```python
from build123d import *

# Parameters (mm, degrees)
SKETCH2_W          = 61.210230612
SKETCH2_H          = 60
EXTRUDE1_DEPTH     = 8
CHAMFER1_SIZE      = 5
SKETCH3_R          = 12
SKETCH3_R_2        = 2.5
CUT_EXTRUDE1_DEPTH = 53.63316445


with BuildPart() as part:
    # Sketch2 → Extrude1 (new body)
    with BuildSketch(Plane(origin=(0, 0, 0), x_dir=(1, 0, 0), z_dir=(0, 1, 0))):
        with Locations((11.894884694, 0)):
            Rectangle(SKETCH2_W, SKETCH2_H)
    extrude(amount=EXTRUDE1_DEPTH)

    # Chamfer1
    chamfer1_edges = [part.edges().sort_by_distance(p)[0] for p in [
        (-18.710230612, 4, 30),
        (-18.710230612, 4, -30),
    ]]
    chamfer(chamfer1_edges, length=CHAMFER1_SIZE)

    # Sketch3 → Cut-Extrude1 (cut, through all)
    with BuildSketch(Plane(origin=(0, 8, 0), x_dir=(1, 0, 0), z_dir=(0, 1, 0))):
        with Locations(Location((12, 0, 0), (0, 0, 270))):
            Circle(SKETCH3_R)
        with Locations(Location((-11.57, 23.57, 0), (0, 0, 270))):
            Circle(SKETCH3_R_2)
        with Locations(Location((35.57, 23.57, 0), (0, 0, 270))):
            Circle(SKETCH3_R_2)
        with Locations(Location((-11.57, -23.57, 0), (0, 0, 270))):
            Circle(SKETCH3_R_2)
        with Locations(Location((35.57, -23.57, 0), (0, 0, 270))):
            Circle(SKETCH3_R_2)
    extrude(amount=-CUT_EXTRUDE1_DEPTH, mode=Mode.SUBTRACT)


solid = part.part
```
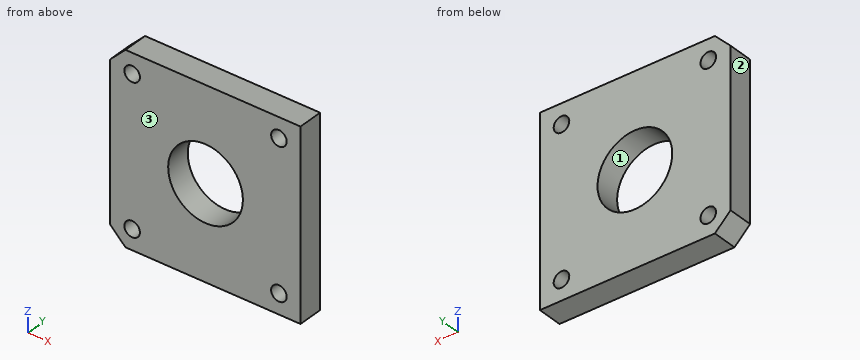
Can you work these out from the model? Positions are in its coordinate system, mm. Face numbers are marked on the shaded views. Coordinates: 2 decimals unless noted, no trailing zeros. Write each loop counter-clockwise with the first axis right and the second up, starting at its lowest first coordinate (ties: lowest second). Pieces come first, ordered by that corner, then holes. Notation, with made-up numbers: M 62.5,-24.75 L 103.5,-24.75 A26 cw 103.5,-4.75 Z; hole C 76.25,12 d8. An arc over 180 degrees is marked long. Answer as CSV lines item,"result".
Item 1: Imagine slicing it at C-C on y = 6.75. List the corners of the cut face in (x, z) for me, plus the area to 3 significant figures.
Geometry results:
outline,"M -18.71,-25 L -13.71,-30 L 42.5,-30 L 42.5,30 L -13.71,30 L -18.71,25 Z; hole C -11.57,-23.57 d5; hole C -11.57,23.57 d5; hole C 12,0 d24; hole C 35.57,-23.57 d5; hole C 35.57,23.57 d5"
area,"3,120 mm2"
Item 2: We'd pull the mould along X, two halves only. Please class the marked faces 1, 2 and 3: +X half, -X half, draft (parallel to the pull), parting line (faces both ways), or undercut.
Geometry results:
face 1,"undercut"
face 2,"-X half"
face 3,"draft"
Item 3: Imagine slicing it at A-A on x = 35.57. List the corners of the cut face in (y, z) for me.
Geometry results:
outline,"M 0,-30 L 8,-30 L 8,-26.07 L 0,-26.07 Z; M 0,-21.07 L 8,-21.07 L 8,21.07 L 0,21.07 Z; M 0,26.07 L 8,26.07 L 8,30 L 0,30 Z"
Item 4: Imagine slicing it at D-D on x = 12. List the corners of the cut face in (y, z) for me.
Geometry results:
outline,"M 0,-30 L 8,-30 L 8,-12 L 0,-12 Z; M 0,12 L 8,12 L 8,30 L 0,30 Z"
Item 5: Imagine slicing it at B-B on z = 23.57. List the corners of the cut face in (x, y) for me.
Geometry results:
outline,"M -18.71,0 L -14.07,0 L -14.07,8 L -18.71,8 Z; M -9.07,0 L 33.07,0 L 33.07,8 L -9.07,8 Z; M 38.07,0 L 42.5,0 L 42.5,8 L 38.07,8 Z"
Item 6: I'm going to push a flat-ended pin straight in: P1, Ø8, axis at x = 35.57, z = -23.57, coming from the +Y side. Where does the tip first touch, or does it pass through?
Geometry results:
P1,"stops at y = 8"
Item 7: Please list where these lines run through material, in increasing order: line 1 along X through (y, z) = (2, -23.57); line 2 along X through (y, z) = (4.25, 0); line 3 along X through (y, z) = (0.5, -22).
Geometry results:
line 1,"x = -18.71 to -14.07, -9.07 to 33.07, 38.07 to 42.5"
line 2,"x = -18.71 to 0, 24 to 42.5"
line 3,"x = -18.71 to -13.52, -9.62 to 33.62, 37.52 to 42.5"
